Build history of the part. All positions in model axes, mm. A direction names the side the tool comes from. Give positions to 0.01 mm unless a question says otherwise; leave off trailing zeros. Write each loop counter-clockwise with the first axis right and the second up, starting at its lowest first coordinate (ties: lowest second). Pieces come first, ordered by that corner, then holes. Notation, with made-up numbers: (28, 70.25) -> (59, 70.25) arc R14 cw to (59, 80.25) -> close; hole circle Ø3 at (74.25, 26.25). An arc over 180 degrees is marked (long way). Write item = value, one per line. Start each with the question number.
Q1. Tool access for faces 1 (the face through (1, 30, 0)), 2 (the face through (0, 1, 9)): list every direction of +Z, -Z, +X, -X, +Y, -Y with a clear straight run to the whole face (end or side of a thin tool).
Q2. Wall check: line 1 (Y direction, x = 1.8, z = -23); line 2 (Y direction, x = 1.5, z = 32.5); line 3 (Y direction, x = 1.15, z = -24). Give the ranges that are in metal, low to high.
Q3. Saw through at D-D, the plane z = -32.5. List the corners of the cut face in (x, y), then the cut area to 3 significant figures.
Q4. Saw through at A-A, the plane y = 41.5. List the corners of the cut face in (x, z), then the cut area to 3 significant figures.
Q5. Saw through at C-C, the plane y = 17.5. List the corners of the cut face in (x, z), then the cut area to 3 significant figures.
Q6. Saw through at B-B, the plane z = 32.5. List the corners of the cut face in (x, y).
from build123d import *

# Parameters (mm, degrees)
SKETCH_1_R          = 1.6
SKETCH_1_R_2        = 10.1
SKETCH_1_R_3        = 2.1
SKETCH_1_R_4        = 7.6
EXTRUDE_1_DEPTH     = 2
SKETCH_3_W          = 50
SKETCH_3_H          = 5
CUT_EXTRUDE_1_DEPTH = 99.508882848
FILLET_1_R          = 3.005
FILLET_2_R          = 2


with BuildPart() as part:
    # ｽｹｯﾁ1 → ﾎﾞｽ - 押し出し1 (new body)
    with BuildSketch(Plane(origin=(0, 0, 0), x_dir=(0, 0, -1), z_dir=(1, 0, 0))):
        with BuildLine():
            Line((-28.07487558, -88.555433417), (36.92512442, -41.055433417))
            ThreePointArc((36.92512442, -41.055433417), (39.187242823, -38.395700727), (40, -35))
            Line((40, -35), (40, 57.5))
            Line((40, 57.5), (-40, 57.5))
            Line((-40, 57.5), (-40, -82.5))
            ThreePointArc((-40, -82.5), (-35.895700727, -89.187242823), (-28.07487558, -88.555433417))
        make_face()
        with Locations((-24.721530862, -67.147937733)):
            Circle(SKETCH_1_R, mode=Mode.SUBTRACT)
        with Locations((-15.529142706, -57.955549577)):
            Circle(SKETCH_1_R_2, mode=Mode.SUBTRACT)
        with Locations((-6.336754551, -67.147937733)):
            Circle(SKETCH_1_R, mode=Mode.SUBTRACT)
        with Locations((-32.5, -35)):
            Circle(SKETCH_1_R_3, mode=Mode.SUBTRACT)
        with Locations((-24.721530862, -48.763161422)):
            Circle(SKETCH_1_R, mode=Mode.SUBTRACT)
        with Locations((-6.336754551, -48.763161422)):
            Circle(SKETCH_1_R, mode=Mode.SUBTRACT)
        with Locations((-15.155444566, -8.75)):
            Circle(SKETCH_1_R, mode=Mode.SUBTRACT)
        with Locations((-32.5, 52.5)):
            Circle(SKETCH_1_R_3, mode=Mode.SUBTRACT)
        Circle(SKETCH_1_R_4, mode=Mode.SUBTRACT)
        with Locations((15.155444566, -8.75)):
            Circle(SKETCH_1_R, mode=Mode.SUBTRACT)
        with Locations((0, 17.5)):
            Circle(SKETCH_1_R, mode=Mode.SUBTRACT)
        with Locations((32.5, 52.5)):
            Circle(SKETCH_1_R_3, mode=Mode.SUBTRACT)
        with Locations((32.5, -35)):
            Circle(SKETCH_1_R_3, mode=Mode.SUBTRACT)
        with Locations((-32.5, -82.5)):
            Circle(SKETCH_1_R_3, mode=Mode.SUBTRACT)
    extrude(amount=EXTRUDE_1_DEPTH)

    # ｽｹｯﾁ3 → ｶｯﾄ - 押し出し1 (cut, through all)
    with BuildSketch(Plane(origin=(2, 0, 0), x_dir=(0, 0, -1), z_dir=(1, 0, 0))):
        with BuildLine():
            Line((25, -31.191591045), (25, -16.583123952))
            ThreePointArc((25, -16.583123952), (0, -30), (-25, -16.583123952))
            Line((-25, -16.583123952), (-25, -40.340134109))
            ThreePointArc((-25, -40.340134109), (-9.984170602, -38.739585267), (1.870513324, -48.093908232))
            Line((1.870513324, -48.093908232), (25, -31.191591045))
        make_face()
        with BuildLine():
            Line((25, 16.583123952), (25, 42.5))
            Line((25, 42.5), (-25, 42.5))
            Line((-25, 42.5), (-25, 16.583123952))
            ThreePointArc((-25, 16.583123952), (0, 30), (25, 16.583123952))
        make_face()
        with Locations((0, 45)):
            Rectangle(SKETCH_3_W, SKETCH_3_H)
    extrude(amount=-CUT_EXTRUDE_1_DEPTH, mode=Mode.SUBTRACT)

    # ﾌｨﾚｯﾄ1
    fillet_1_edges = [part.edges().sort_by_distance(p)[0] for p in [
        (1, -48.093908232, -1.870513324),
        (1, -40.340134109, 25),
        (1, -16.583123952, 25),
        (1, -16.583123952, -25),
        (1, -31.191591045, -25),
        (1, 16.583123952, -25),
        (1, 16.583123952, 25),
        (1, 47.5, 25),
        (1, 47.5, -25),
    ]]
    fillet(fillet_1_edges, radius=FILLET_1_R)

    # ﾌｨﾚｯﾄ2
    fillet_2_edges = [part.edges().sort_by_distance(p)[0] for p in [
        (1, 57.5, 40),
        (1, 57.5, -40),
    ]]
    fillet(fillet_2_edges, radius=FILLET_2_R)


solid = part.part
Report:
q1.face_1 = +X, -X
q1.face_2 = +Z, -Z, -X, +Y, -Y
q2.line_1 = -51.23 to -32.65, -21.78 to 21.78, 47.33 to 57.5
q2.line_2 = -90 to -84.6, -80.4 to -37.1, -32.9 to 50.4, 54.6 to 57.5
q2.line_3 = -50.5 to -31.9, -22.37 to 22.37, 46.73 to 57.5
q3.outline = (0, -44.29) -> (2, -44.29) -> (2, -37.1) -> (0, -37.1) -> close; (0, -32.9) -> (2, -32.9) -> (2, 50.4) -> (0, 50.4) -> close; (0, 54.6) -> (2, 54.6) -> (2, 57.5) -> (0, 57.5) -> close
q3.area = 187 mm2
q4.outline = (0, -40) -> (2, -40) -> (2, -25) -> (0, -25) -> close; (0, 25) -> (2, 25) -> (2, 40) -> (0, 40) -> close
q4.area = 60.0 mm2
q5.outline = (0, -40) -> (2, -40) -> (2, -1.6) -> (0, -1.6) -> close; (0, 1.6) -> (2, 1.6) -> (2, 40) -> (0, 40) -> close
q5.area = 154 mm2
q6.outline = (0, -90) -> (2, -90) -> (2, -84.6) -> (0, -84.6) -> close; (0, -80.4) -> (2, -80.4) -> (2, -37.1) -> (0, -37.1) -> close; (0, -32.9) -> (2, -32.9) -> (2, 50.4) -> (0, 50.4) -> close; (0, 54.6) -> (2, 54.6) -> (2, 57.5) -> (0, 57.5) -> close
